```python
from build123d import *

# Parameters (mm, degrees)
BOSS_EXTRUDE1_DEPTH     = 25
CUT_EXTRUDE2_DEPTH      = 110.201648339
CUT_EXTRUDE2_DEPTH_BACK = 110.201648339
SKETCH2_W               = 45
SKETCH2_H               = 12
CHAMFER1_SIZE           = 8
SKETCH3_R               = 7.5
SKETCH3_R_2             = 4
CUT_EXTRUDE3_DEPTH      = 25
SKETCH4_R               = 12.5
CUT_EXTRUDE4_DEPTH      = 5
SKETCH5_W               = 4
SKETCH5_H               = 52.762109512
CUT_EXTRUDE5_DEPTH      = 110.201648339
SKETCH6_R               = 7.5
CUT_EXTRUDE6_DEPTH      = 15


with BuildPart() as part:
    # Sketch1 → Boss-Extrude1 (new body)
    with BuildSketch(Plane(origin=(0, 0, 0), x_dir=(1, 0, 0), z_dir=(0, 1, 0))):
        Polygon((25, 0), (55, 0), (55, 15), (80, 15), (80, 70), (0, 70), (0, 15), (25, 15), align=None)
    extrude(amount=BOSS_EXTRUDE1_DEPTH)

    # Sketch2 → Cut-Extrude2 (cut, two sides: drawn at the far end of the back side and taken through both)
    with BuildSketch(Plane(origin=(0, 0, 0), x_dir=(0, 0, -1), z_dir=(1, 0, 0)).offset(-CUT_EXTRUDE2_DEPTH_BACK)):
        with Locations((47.5, 19)):
            Rectangle(SKETCH2_W, SKETCH2_H)
    extrude(amount=CUT_EXTRUDE2_DEPTH + CUT_EXTRUDE2_DEPTH_BACK, mode=Mode.SUBTRACT)

    # Chamfer1
    chamfer1_edges = [part.edges().sort_by_distance(p)[0] for p in [
        (40, 0, -70),
    ]]
    chamfer(chamfer1_edges, length=CHAMFER1_SIZE)

    # Sketch3 → Cut-Extrude3 (cut)
    with BuildSketch(Plane(origin=(0, 13, 0), x_dir=(1, 0, 0), z_dir=(0, 1, 0))):
        with Locations(Location((40, 50, 0), (0, 0, 270))):
            Circle(SKETCH3_R)
        with Locations(Location((65, 50, 0), (0, 0, 270))):
            Circle(SKETCH3_R_2)
        with Locations(Location((15, 50, 0), (0, 0, 270))):
            Circle(SKETCH3_R_2)
    extrude(amount=-CUT_EXTRUDE3_DEPTH, mode=Mode.SUBTRACT)

    # Sketch4 → Cut-Extrude4 (cut)
    with BuildSketch(Plane(origin=(0, 13, 0), x_dir=(1, 0, 0), z_dir=(0, 1, 0))):
        with Locations(Location((40, 50, 0), (0, 0, 270))):
            Circle(SKETCH4_R)
    extrude(amount=-CUT_EXTRUDE4_DEPTH, mode=Mode.SUBTRACT)

    # Sketch5 → Cut-Extrude5 (cut, through all)
    with BuildSketch(Plane(origin=(0, 25, 0), x_dir=(1, 0, 0), z_dir=(0, 1, 0))):
        with Locations((40, 25.178276377)):
            Rectangle(SKETCH5_W, SKETCH5_H)
    extrude(amount=-CUT_EXTRUDE5_DEPTH, mode=Mode.SUBTRACT)

    # Sketch6 → Cut-Extrude6 (cut)
    with BuildSketch(Plane.XY):
        with Locations((40, 13)):
            Circle(SKETCH6_R)
    extrude(amount=-CUT_EXTRUDE6_DEPTH, mode=Mode.SUBTRACT)


solid = part.part
```
Here's how the part is built. I have some questions about the finished solid (model axes, mm). A direction names the side the tool comes from. Give positions to 0.01 mm unless a question says otherwise; leave off trailing zeros. Loops run counter-clockwise (first coordinate to the right, second up) from the corner with the lowest first, then second, coordinate; pieces in that order, holes last. Notation, with made-up numbers: M 64.5,47.5 L 102.5,47.5 A12 ccw 102.5,64.5 Z; hole C 47.25,6 d4. An arc over 180 degrees is marked long. Return JSON: item names as keys, results as strings.
Item 1: Please list where these lines run through material, in increasing order: line 1 (X direction, y = 4.25, z = -50); line 2 (X direction, y = 9.55, z = -50); line 3 (X direction, y = 2, z = -41.5).
A:
{"line 1": "x = 0 to 11, 19 to 32.5, 47.5 to 61, 69 to 80", "line 2": "x = 0 to 11, 19 to 27.5, 52.5 to 61, 69 to 80", "line 3": "x = 0 to 38, 42 to 80"}
Item 2: Imagine slicing it at D-D on z = -50. List the corners of the cut face in (x, y) for me.
A:
{"outline": "M 0,0 L 11,0 L 11,13 L 0,13 Z; M 19,0 L 32.5,0 L 32.5,8 L 27.5,8 L 27.5,13 L 19,13 Z; M 47.5,0 L 61,0 L 61,13 L 52.5,13 L 52.5,8 L 47.5,8 Z; M 69,0 L 80,0 L 80,13 L 69,13 Z"}
Item 3: On a 3-axis mill with a long thin cutter (end or side, diameter ignored), from which of +Z, -Z, +X, -X, +Y, -Y can I reach the whole of each face in a straight line? I mean faces 5 (the flat face through (38, 10, -21)), 6 (the cylindrical face through (40.52, 10.54, -62.49)), 7 (the flat face through (61, 19, -25)). Say none if no direction works.
A:
{"face 5": "+Z, +Y, -Y", "face 6": "+Y", "face 7": "-Z, +X, -X, +Y"}
Item 4: Imagine slicing it at B-B on x = 65. List the corners of the cut face in (y, z) for me.
A:
{"outline": "M 0,-62 L 8,-70 L 13,-70 L 13,-54 L 0,-54 Z; M 0,-46 L 13,-46 L 13,-25 L 25,-25 L 25,-15 L 0,-15 Z"}
Item 5: Imagine slicing it at C-C on y = 2. List the corners of the cut face in (x, z) for me, then the cut area to 3 significant figures.
A:
{"outline": "M 0,-64 L 80,-64 L 80,-15 L 55,-15 L 55,0 L 42,0 L 42,-42.77 A7.5 cw long 38,-42.77 L 38,0 L 25,0 L 25,-15 L 0,-15 Z; hole C 15,-50 d8; hole C 65,-50 d8", "area": "3,920 mm^2"}
Item 6: Imagine slicing it at A-A on z = -35.5. List the corners of the cut face in (x, y) for me, then the cut area to 3 significant figures.
A:
{"outline": "M 0,0 L 38,0 L 38,13 L 0,13 Z; M 42,0 L 80,0 L 80,13 L 42,13 Z", "area": "988 mm^2"}
Item 7: I'm going to push flat-ended pins straight in: pin 1 Ø12 at (y, z) = (6.5, -43.5) entering from -X; pin 2 Ø9 at (x, z) = (40, -50) entering from +Y; pin 3 Ø9 at (x, z) = (65, -50) entering from +Y; pin 4 Ø12 at (y, z) = (14, -6) entering from +X. Where does each tip first touch, or does it pass through?
A:
{"pin 1": "stops at x = 0", "pin 2": "passes through", "pin 3": "stops at y = 13", "pin 4": "stops at x = 55"}
Item 8: Thinking about a two-plate mould opening in Z: for faces 1 (the flat face through (25, 12, -8)), 2 (the cylindrical face through (17.7, 6.59, -52.95)), 3 (the cylindrical face through (61.095, 6.591, -50.867)), 4 (the flat face through (41, 10, -70)), which applies, released by +Z, released by -Z, zero draft, split by the parting line, or undercut?
A:
{"face 1": "zero draft", "face 2": "undercut", "face 3": "undercut", "face 4": "released by -Z"}
